from build123d import *

# Parameters (mm, degrees)
F1_DEPTH = 5


with BuildPart() as f1:
    # F0 (on Top) → F1 (new body)
    with BuildSketch(Plane.XY):
        Polygon((5, 0), (0, 0), (-5, 0), (-7, 0), (-7, -2), (0, -2), (7, -2), (7, 0), align=None)
        Polygon((5, 20), (5, 0), (7, 0), (25, 0), (25, 18), (25, 20), (23, 20), align=None)
        Polygon((-7, 0), (-5, 0), (-5, 20), (-23, 20), (-25, 20), (-25, 18), (-25, 0), align=None)
        Polygon((23, 22), (23, 20), (25, 20), (25, 18), (27, 18), (27, 22), align=None)
        Polygon((-25, 20), (-23, 20), (-23, 22), (-27, 22), (-27, 18), (-25, 18), align=None)
    extrude(amount=F1_DEPTH)


solid = f1.part
Read the model definition and answer for the solid it produces. Units are mm, in the model's axes. A direction names the side the tool comes from. Coordinates: 2 decimals unless noted, no trailing zeros. Loops run counter-clockwise (first coordinate to the right, second up) from the corner with the lowest first, then second, coordinate; pieces in that order, holes last. Notation, with made-up numbers: (-10, 0.5) -> (9, 0.5) arc R21 cw to (9, 7.5) -> close; hole circle Ø10 at (10, -23.5). An arc over 180 degrees is marked (long way). Write item = value, one per line. Start each with the question number.
1) The part is cut by section B-B, the plane z = 1.05. Determine the outline of the cut face in (x, y).
2) Find the intervals of material crossed by L1, parallel to X at y = 10, z = 4.35; L2, parallel to X at y = 20.75, z = 4.55; L3, parallel to Y at x = -22.5, z = 0.7, in increasing order. Write a range as from..to.
3) The mould has two halves that part along X. Classify faces 4 (the face through (-26, 18, 2)), 5 (the face through (-5, 10, 2)), 6 (the face through (25, 9, 2)): pulls with the +X half, pulls with the -X half, needs draft (parallel to the pull), parting line crosses it, or undercut.
4) Given P1, Ø10, axis at x = -17.5, y = 12, coming from the -Z side; P2, Ø1.6, axis at y = -0.5, z = 1.5, coming from the -X side; P3, Ø0.6, axis at x = -26, z = 1.5, coming from the -Y side; P4, Ø1.5, axis at x = -2, z = 3, coming from the +Y side, each flat-ended and moving along its own axis, determine where each tip first touches the part or whether it passes through.
5) The part is cut by section A-A, the plane y = 12.25. Determine the outline of the cut face in (x, z), plus the area to 3 significant figures.
6) The part is cut by section C-C, the plane x = 12. Determine the outline of the cut face in (y, z), plus the area to 3 significant figures.
7) For faces 1 (the face through (-25, 9, 2)), 2 (the face through (-23, 21, 2)), 3 (the face through (26, 18, 2)), determine the directions among +Z, -Z, +X, -X, +Y, -Y from which every point of the face is accessible in a straight line to the end or side of a thin tool.
Result:
q1.outline = (-27, 18) -> (-25, 18) -> (-25, 0) -> (-7, 0) -> (-7, -2) -> (7, -2) -> (7, 0) -> (25, 0) -> (25, 18) -> (27, 18) -> (27, 22) -> (23, 22) -> (23, 20) -> (5, 20) -> (5, 0) -> (-5, 0) -> (-5, 20) -> (-23, 20) -> (-23, 22) -> (-27, 22) -> close
q2.L1 = -25..-5, 5..25
q2.L2 = -27..-23, 23..27
q2.L3 = 0..20
q3.face_4 = needs draft
q3.face_5 = undercut
q3.face_6 = pulls with the +X half
q4.P1 = 0
q4.P2 = -25
q4.P3 = 18
q4.P4 = 0
q5.outline = (-25, 0) -> (-5, 0) -> (-5, 5) -> (-25, 5) -> close; (5, 0) -> (25, 0) -> (25, 5) -> (5, 5) -> close
q5.area = 200 mm²
q6.outline = (0, 0) -> (20, 0) -> (20, 5) -> (0, 5) -> close
q6.area = 100 mm²
q7.face_1 = +Z, -Z, -X, -Y
q7.face_2 = +Z, -Z, +Y
q7.face_3 = +Z, -Z, +X, -Y
